Build history of the part. All positions in model axes, mm. Face numbers are marked on the shaded views. A direction names the side the tool comes from. Round coordinates to 2 decimals unless told otherwise and drop trailing zeros. Loops run counter-clockwise (first coordinate to the right, second up) from the corner with the lowest first, then second, coordinate; pieces in that order, holes last. Notation, with made-up numbers: (-39.5, 69) -> (15.5, 69) arc R15 ccw to (15.5, 94) -> close; hole circle Ø3 at (27.25, 57.25). An arc over 180 degrees is marked (long way). Put each result on its own line as item: value. Start each with the question number.
Item 1: Pull direction Y, two halves, no side cores. Call the marked faces 1, 2 and 3: +Y half, -Y half, draft (parallel to the pull), parting line (faces both ways), or undercut.
Item 2: Flat gauge pins, fed straight in: pin 1 Ø6 at (x, z) = (144, 21) entering from -Y; pin 2 Ø9 at (y, z) = (-24, 23) entering from -X; pin 3 Ø12 at (x, y) = (53.5, -36) entering from +Z. Where does each tip first touch, or does it go through?
Item 3: Cut at A-A, the plane z = 38.1. Count the separate pieces of the cut face and the enclosed holes in it, plus the area to 3 significant figures.
Item 4: Cut at B-B, the plane z = 20. List the corners of the cut face in (x, y) (3 decimals), plus the area to 3 significant figures.
Item 5: Cut at C-C, the plane x = 50.8. List the corners of the cut face in (y, z) (3 decimals), plus the area to 3 significant figures.
Item 6: Cut at D-D, the plane y = -27.94. List the corners of the cut face in (x, z) (3 decimals).
Item 7: Tool access for the marked faces 4, 5 and 6: list every direction of +Z, -Z, +X, -X, +Y, -Y with a clear straight run to the whole face (end or side of a thin tool).
Item 8: Drill centre lines: probe 1 along X at (y, z) = (-27, 37); probe 2 along X at (y, z) = (-15.5, 37.5); probe 3 along Y at (x, z) = (96, 24) (3 decimals). Where is each one in solid material? Low to high. Write a range as [from, to].
```python
from build123d import *

# Parameters (mm, degrees)
F0_W     = 25.4
F0_H     = 50.8
F0_R     = 2.54
F0_W_2   = 50.8
F1_DEPTH = 6.35
F2_DEPTH = 52.705
F3_R     = 5.08
F4_R     = 20.955
F5_DEPTH = 44.45
F6_R     = 22.86
F7_SIZE  = 0.762


with BuildPart() as f1:
    # F0 (on Front) → F1 (new body)
    with BuildSketch(Plane.XZ):
        with Locations((12.7, 25.4)):
            Rectangle(F0_W, F0_H)
        with Locations((9.652, 12.7)):
            Circle(F0_R, mode=Mode.SUBTRACT)
        with Locations((9.652, 38.1)):
            Circle(F0_R, mode=Mode.SUBTRACT)
        with Locations((139.7, 25.4)):
            Rectangle(F0_W, F0_H)
        with Locations((142.748, 12.7)):
            Circle(F0_R, mode=Mode.SUBTRACT)
        with Locations((142.748, 38.1)):
            Circle(F0_R, mode=Mode.SUBTRACT)
        with Locations((50.8, 25.4)):
            Rectangle(F0_W_2, F0_H)
        with Locations((101.6, 25.4)):
            Rectangle(F0_W_2, F0_H)
    extrude(amount=F1_DEPTH)

    # F0 (on Front) → F2 (join)
    with BuildSketch(Plane.XZ):
        with Locations((50.8, 25.4)):
            Rectangle(F0_W_2, F0_H)
        with Locations((101.6, 25.4)):
            Rectangle(F0_W_2, F0_H)
    extrude(amount=F2_DEPTH)

    # F3
    f3_edges = [f1.edges().sort_by_distance(p)[0] for p in [
        (127, -6.35, 25.4),
        (25.4, -6.35, 25.4),
    ]]
    fillet(f3_edges, radius=F3_R)

    # F4 (on face) → F5 (cut)
    with BuildSketch(Plane.XY.offset(50.8)):
        with Locations((50.8, -27.94)):
            Circle(F4_R)
        with Locations((101.6, -27.94)):
            Circle(F4_R)
    extrude(amount=-F5_DEPTH, mode=Mode.SUBTRACT)

    # F6
    f6_edges = [f1.edges().sort_by_distance(p)[0] for p in [
        (127, -52.705, 25.4),
        (25.4, -52.705, 25.4),
    ]]
    fillet(f6_edges, radius=F6_R)

    # F7
    f7_edges = [f1.edges().sort_by_distance(p)[0] for p in [
        (127, -20.6375, 50.8),
        (120.304461, -46.009461, 50.8),
        (128.487898, -7.837898, 50.8),
        (76.2, -52.705, 50.8),
        (142.24, -6.35, 50.8),
        (32.095539, -46.009461, 50.8),
        (152.4, -3.175, 50.8),
        (25.4, -20.6375, 50.8),
        (76.2, 0, 50.8),
        (23.912102, -7.837898, 50.8),
        (0, -3.175, 50.8),
        (10.16, -6.35, 50.8),
        (80.645, -27.94, 50.8),
        (29.845, -27.94, 50.8),
        (20.32, -6.35, 25.4),
        (0, -6.35, 25.4),
        (10.16, -6.35, 0),
        (7.112, -6.35, 12.7),
        (7.112, -6.35, 38.1),
        (132.08, -6.35, 25.4),
        (152.4, -6.35, 25.4),
        (142.24, -6.35, 0),
        (140.208, -6.35, 12.7),
        (140.208, -6.35, 38.1),
        (25.4, -20.6375, 0),
        (32.095539, -46.009461, 0),
        (23.912102, -7.837898, 0),
        (76.2, -52.705, 0),
        (120.304461, -46.009461, 0),
        (0, -3.175, 0),
        (127, -20.6375, 0),
        (76.2, 0, 0),
        (128.487898, -7.837898, 0),
        (152.4, -3.175, 0),
        (0, 0, 25.4),
        (152.4, 0, 25.4),
        (7.112, 0, 12.7),
        (7.112, 0, 38.1),
        (140.208, 0, 38.1),
        (140.208, 0, 12.7),
        (29.845, -27.94, 6.35),
        (80.645, -27.94, 6.35),
    ]]
    chamfer(f7_edges, length=F7_SIZE)


solid = f1.part
```
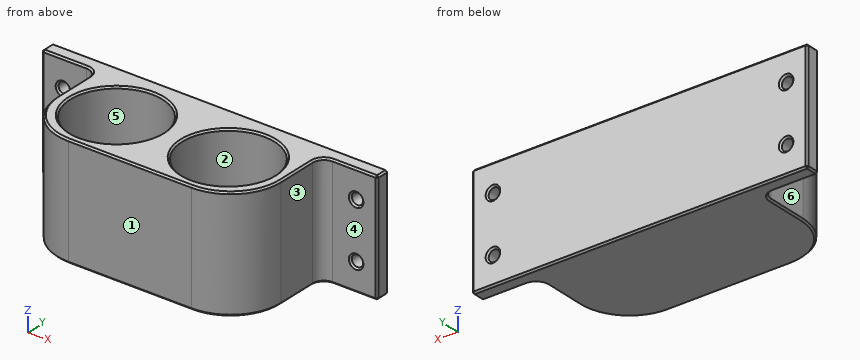
Reply:
1. face 1: -Y half
1. face 2: undercut
1. face 3: draft
2. pin 1: stops at y = -6.35
2. pin 2: stops at x = 25.4
2. pin 3: stops at z = 6.35
3. separate pieces: 3
3. enclosed holes: 2
3. area: 2,640 mm^2
4. outline: (0, -5.588) -> (0.762, -6.35) -> (20.32, -6.35) arc R5.08 cw to (25.4, -11.43) -> (25.4, -29.845) arc R22.86 ccw to (48.26, -52.705) -> (104.14, -52.705) arc R22.86 ccw to (127, -29.845) -> (127, -11.43) arc R5.08 cw to (132.08, -6.35) -> (151.638, -6.35) -> (152.4, -5.588) -> (152.4, -0.762) -> (151.638, 0) -> (0.762, 0) -> (0, -0.762) -> close; hole circle Ø41.91 at (50.8, -27.94); hole circle Ø41.91 at (101.6, -27.94)
4. area: 2,700 mm^2
5. outline: (-52.705, 0.762) -> (-51.943, 0) -> (-0.762, 0) -> (0, 0.762) -> (0, 50.038) -> (-0.762, 50.8) -> (-6.223, 50.8) -> (-6.985, 50.038) -> (-6.985, 7.112) -> (-7.747, 6.35) -> (-48.133, 6.35) -> (-48.895, 7.112) -> (-48.895, 50.038) -> (-49.657, 50.8) -> (-51.943, 50.8) -> (-52.705, 50.038) -> close
5. area: 813 mm^2
6. outline: (25.4, 0.762) -> (26.162, 0) -> (126.238, 0) -> (127, 0.762) -> (127, 50.038) -> (126.238, 50.8) -> (123.317, 50.8) -> (122.555, 50.038) -> (122.555, 7.112) -> (121.793, 6.35) -> (81.407, 6.35) -> (80.645, 7.112) -> (80.645, 50.038) -> (79.883, 50.8) -> (72.517, 50.8) -> (71.755, 50.038) -> (71.755, 7.112) -> (70.993, 6.35) -> (30.607, 6.35) -> (29.845, 7.112) -> (29.845, 50.038) -> (29.083, 50.8) -> (26.162, 50.8) -> (25.4, 50.038) -> close
7. face 4: +Z, -Z, +X, -Y
7. face 5: +Z
7. face 6: +Z, -Z, -X, -Y
8. probe 1: x = [25.4, 29.87], [71.73, 80.67], [122.53, 127]
8. probe 2: x = [25.4, 33.94], [67.66, 84.74], [118.46, 127]
8. probe 3: y = [-52.705, -48.133], [-7.747, 0]
